Geometry check sheet. Reference: the model listing, model coordinates, mm. A direction names the side the tool comes from. Round coordinates to 2 decimals unless told otherwise and drop trailing zeros. Loops run counter-clockwise (first coordinate to the right, second up) from the corner with the lowest first, then second, coordinate; pieces in that order, holes last. Notation, with made-up numbers: (83, 87) - (119, 87) arc R22 cw to (119, 103) - close; hole circle Ø7 at (34, 39.5). An arc over 180 degrees is marked (long way). Answer as CSV lines item,"result". Start each with the question number.
1) Cross-section at C-C on x = -1.5. Record the boundary of the cut face in (y, z).
2) Thickness scan on line 1 along Z through (x, y) = (0, -16.7); line 2 along Y through (x, z) = (0, -2.7); line 3 along Y through (x, z) = (-10.5, -5). Record the ranges inside material, lowest first.
3) Access from +Z, -Z, +X, -X, +Y, -Y to the whole of each face (thin tool, end or side, straight path). Record for faces 4 (the flat face through (7, -15, 0)), 5 (the cylindrical face through (-9.4, -16.5, -1.2)).
4) Depth check by flat-ended pin: P1, Ø10, axis at y = -5.5, z = -1.5, coming from the -X side; P2, Ø6, axis at x = 4.5, y = -8, coming from the -Z side; P3, Ø1, axis at x = 2, y = -6, coming from the +Z side. Enter the tip coordinate at first touch or a pass-through.
5) Draft check along X on faces 1 (the cylindrical face through (5.08, -7.4, 2.11)), 2 (the cylindrical face through (12.6, -16.5, -1.2)), 3 (the flat face through (-3, 0, 0)). Enter one of: released by +X, released by -X, zero draft, split by the parting line, or undercut.
6) Cross-section at D-D on z = -1. Record the boundary of the cut face in (x, y), and give its area (3 significant figures).
7) Cross-section at A-A on y = -3.25. Record the boundary of the cut face in (x, z).
8) Cross-section at B-B on z = -10. Record the boundary of the cut face in (x, y).
from build123d import *

# Parameters (mm, degrees)
CUT_EXTRUDE1_DEPTH      = 10
CUT_EXTRUDE1_DEPTH_BACK = 10
SKETCH2_R               = 2
SKETCH3_R               = 2
CUT_EXTRUDE2_DEPTH      = 10


with BuildPart() as part:
    # Sketch1 → Revolve1 (revolve)
    with BuildSketch(Plane.XY, mode=Mode.PRIVATE) as revolve1_sk:
        Polygon((-2.5, 0), (-2.5, -18), (-15.5, -18), (-15.5, -15), (-5.5, -15), (-5.5, 0), align=None)
    revolve(revolve1_sk.sketch.rotate(Axis((0, -76.950705693, 0), (0, 1, 0)), 180), axis=Axis((0, -76.950705693, 0), (0, 1, 0)))

    # Sketch2 → Cut-Extrude1 (cut, two sides: drawn at the far end of the back side and taken through both)
    with BuildSketch(Plane.XY.offset(-CUT_EXTRUDE1_DEPTH_BACK)):
        with Locations(Location((0, -4.46288306, 0), (0, 0, 180))):
            Circle(SKETCH2_R)
    extrude(amount=CUT_EXTRUDE1_DEPTH + CUT_EXTRUDE1_DEPTH_BACK, mode=Mode.SUBTRACT)

    # Sketch3 → Cut-Extrude2 (cut)
    with BuildSketch(Plane(origin=(0, -15, 0), x_dir=(1, 0, 0), z_dir=(0, 1, 0))):
        with Locations(Location((0, 11, 0), (0, 0, 180))):
            Circle(SKETCH3_R)
        with Locations(Location((11, 0, 0), (0, 0, 180))):
            Circle(SKETCH3_R)
        with Locations(Location((0, -11, 0), (0, 0, 180))):
            Circle(SKETCH3_R)
        with Locations(Location((-11, 0, 0), (0, 0, 180))):
            Circle(SKETCH3_R)
    extrude(amount=-CUT_EXTRUDE2_DEPTH, mode=Mode.SUBTRACT)


solid = part.part
Answer block:
1,outline,"(-18, -15.43) - (-15, -15.43) - (-15, -12.32) - (-18, -12.32) - close; (-18, -9.68) - (-15, -9.68) - (-15, -5.29) - (-5.79, -5.29) - (-5.79, -2) - (-18, -2) - close; (-18, 2) - (-5.79, 2) - (-5.79, 5.29) - (-15, 5.29) - (-15, 9.68) - (-18, 9.68) - close; (-18, 12.32) - (-15, 12.32) - (-15, 15.43) - (-18, 15.43) - close; (-3.14, -5.29) - (0, -5.29) - (0, -2) - (-3.14, -2) - close; (-3.14, 2) - (0, 2) - (0, 5.29) - (-3.14, 5.29) - close"
2,line 1,"z = -15.5 to -13, -9 to -2.5, 2.5 to 9, 13 to 15.5"
2,line 2,"y = -18 to -6.46, -2.46 to 0"
2,line 3,"y = -18 to -15"
3,face 4,"+Y"
3,face 5,"+Y, -Y"
4,P1,"stops at x = -5.5"
4,P2,"stops at z = -5.29"
4,P3,"stops at z = 5.29"
5,face 1,"split by the parting line"
5,face 2,"undercut"
5,face 3,"zero draft"
6,outline,"(-15.47, -18) - (-12.73, -18) - (-12.73, -15) - (-15.47, -15) - close; (-9.27, -18) - (-2.29, -18) - (-2.29, 0) - (-5.41, 0) - (-5.41, -15) - (-9.27, -15) - close; (2.29, -18) - (9.27, -18) - (9.27, -15) - (5.41, -15) - (5.41, 0) - (2.29, 0) - close; (12.73, -18) - (15.47, -18) - (15.47, -15) - (12.73, -15) - close"
6,area,"152 mm^2"
7,outline,"(-1.59, -5.27) - (-1.59, -1.93) arc R2.5 cw to (-1.59, 1.93) - (-1.59, 5.27) arc R5.5 ccw to start; (1.59, -5.27) arc R5.5 ccw to (1.59, 5.27) - (1.59, 1.93) arc R2.5 cw to (1.59, -1.93) - close"
8,outline,"(-11.84, -18) - (-1.73, -18) - (-1.73, -15) - (-11.84, -15) - close; (1.73, -18) - (11.84, -18) - (11.84, -15) - (1.73, -15) - close"
